Geometry check sheet. Reference: the model listing, model coordinates, mm. Coordinates: 2 decimals unless noted, no trailing zeros.
from build123d import *

# Parameters (mm, degrees)
ESQUISSE1_W        = 7.3
ESQUISSE1_H        = 7.3
ESQUISSE1_R        = 2.15
BOSS_EXTRU_2_DEPTH = 600


with BuildPart() as part:
    # Esquisse1 → Boss.-Extru.2 (new body)
    with BuildSketch(Plane.XY):
        Polygon((-8, -2.5), (-10, -2.5), (-10, -10), (-2.5, -10), (-2.5, -8), (-6.585786438, -8), (-2.235786438, -3.65), (-3.65, -3.65), (-3.65, -2.235786438), (-8, -6.585786438), align=None)
        Polygon((2.5, -8), (2.5, -10), (10, -10), (10, -8), (9.414213562, -8), (8, -6.585786438), (3.65, -2.235786438), (3.65, -3.65), (2.235786438, -3.65), (6.585786438, -8), align=None)
        Rectangle(ESQUISSE1_W, ESQUISSE1_H)
        Circle(ESQUISSE1_R, mode=Mode.SUBTRACT)
        Polygon((10, 10), (2.5, 10), (2.5, 8), (6.585786438, 8), (2.235786438, 3.65), (3.65, 3.65), (3.65, 2.235786438), (8, 6.585786438), (9.414213562, 8), (10, 8), align=None)
        Polygon((17.5, 10), (10, 10), (10, 8), (10.585786438, 8), (12, 6.585786438), (16.35, 2.235786438), (16.35, 3.65), (17.764213562, 3.65), (13.414213562, 8), (17.5, 8), align=None)
        Polygon((-2.5, 10), (-10, 10), (-10, 2.5), (-8, 2.5), (-8, 6.585786438), (-3.65, 2.235786438), (-3.65, 3.65), (-2.235786438, 3.65), (-6.585786438, 8), (-2.5, 8), align=None)
        Polygon((10, -8), (10, -10), (17.5, -10), (17.5, -8), (13.414213562, -8), (17.764213562, -3.65), (16.35, -3.65), (16.35, -2.235786438), (12, -6.585786438), (10.585786438, -8), align=None)
        Polygon((22.235786438, 3.65), (17.764213562, 3.65), (16.35, 3.65), (16.35, 2.235786438), (16.35, -2.235786438), (16.35, -3.65), (17.764213562, -3.65), (22.235786438, -3.65), (23.65, -3.65), (23.65, -2.235786438), (23.65, 2.235786438), (23.65, 3.65), align=None)
        with Locations((20, 0)):
            Circle(ESQUISSE1_R, mode=Mode.SUBTRACT)
        Polygon((30, 10), (22.5, 10), (22.5, 8), (26.585786438, 8), (22.235786438, 3.65), (23.65, 3.65), (23.65, 2.235786438), (28, 6.585786438), (28, 2.5), (30, 2.5), align=None)
        Polygon((30, -10), (30, -2.5), (28, -2.5), (28, -6.585786438), (23.65, -2.235786438), (23.65, -3.65), (22.235786438, -3.65), (26.585786438, -8), (22.5, -8), (22.5, -10), align=None)
    extrude(amount=BOSS_EXTRU_2_DEPTH)


solid = part.part
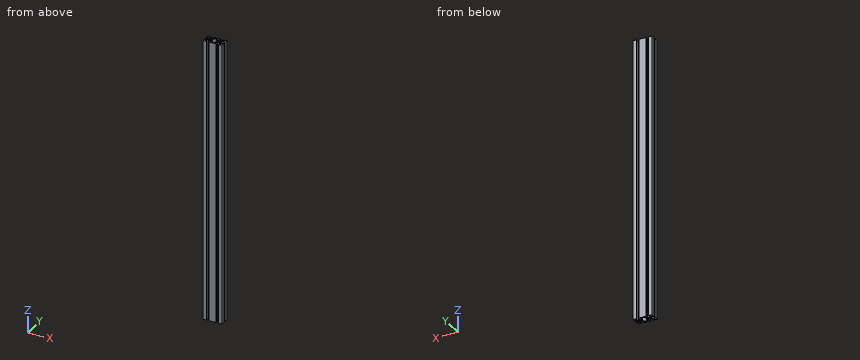
1. Thickness scan on line 1 along X through (y, z) = (-0.25, 211.5); line 2 along Y through (x, z) = (9.5, 259.5); line 3 along Y through (x, z) = (0, 380.5). Record the ranges inside material, lowest first.
Computed values:
line 1: x = -3.65 to -2.14, 2.14 to 3.65, 16.35 to 17.86, 22.14 to 23.65
line 2: y = -10 to -8, 8 to 10
line 3: y = -3.65 to -2.15, 2.15 to 3.65
2. Sectioned sample at A-A, the plane z = 505. Give the number of separate pieces and of enclosed holes in the cut face, and give its area (3 significant figures).
Computed values:
separate pieces: 1
enclosed holes: 3
area: 344 mm2
3. Gauge pin test, flat ends, axial feed: pin 1 Ø5 at (y, z) = (-1, 309) entering from -X; pin 2 Ø2 at (y, z) = (-1, 363) entering from +X; pin 3 Ø2 at (x, z) = (19.5, 239) entering from +Y. Record the tip position at first contact, or that the pin passes through.
Computed values:
pin 1: stops at x = -10
pin 2: stops at x = 23.65
pin 3: stops at y = 3.65
